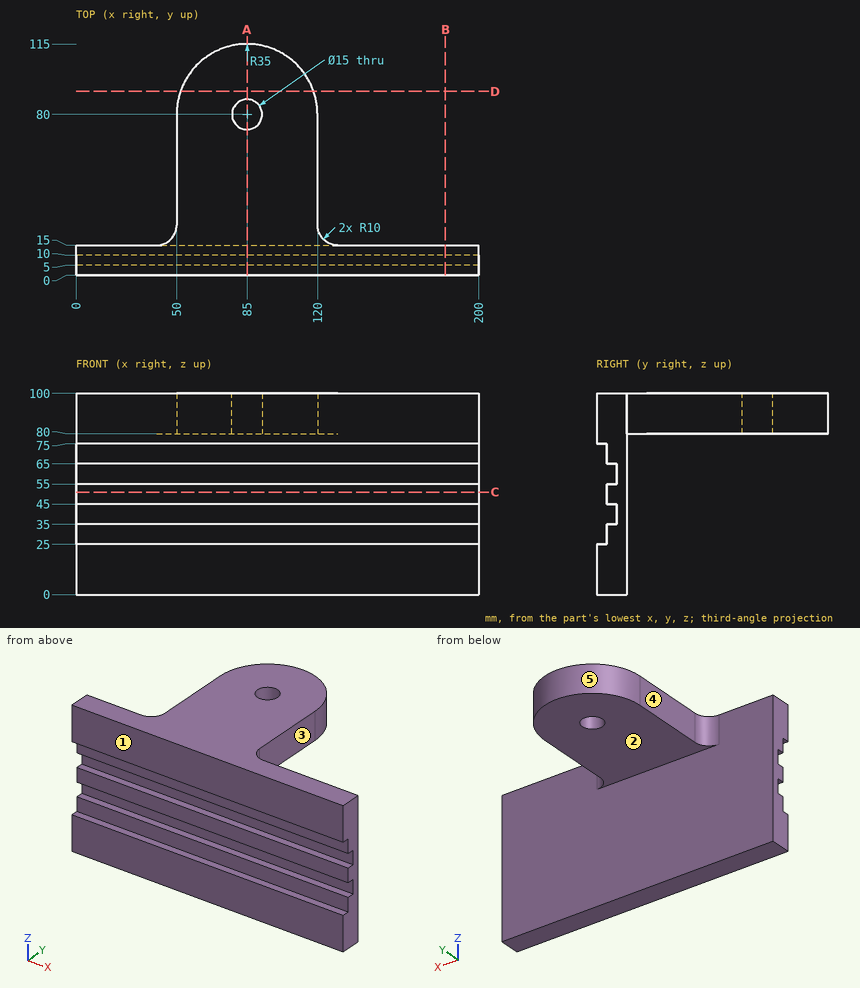
Print and shaded views of the part. All mm, measured from the part's lowest x, y and z. A direction names the side the tool comes from. Round coordinates to 2 decimals unless told otherwise and drop trailing zeros. Write each loop counter-clockwise with the first axis right and the second up, starting at its lowest first coordinate (ties: lowest second). Pieces come first, ordered by that corner, then holes. Notation, with made-up numbers: (2, 72) - (38, 72) arc R22 ccw to (38, 110) - close; hole circle Ø6 at (1, -13). An arc over 180 degrees is marked (long way). Write each question's results on one line, items separated by ' | '. Start each with the question number.
Item 1: Which spindle directions (+Z, -Z, +X, -X, +Y, -Y) get a long thin tool onto all of the face, cutting with end or side? Do the marked faces 1, 2, 3, 4 and 5. Say none if no direction does.
Item 2: Saw through at D-D (y = 91.5). Write the cut outline in (x, z).
Item 3: Drop flat-ended pins along their axis: P1, Ø8, axis at x = 112.5, z = 48.5, coming from the -Y side; P2, Ø8, axis at x = 59, y = 65, coming from the -Z side; P3, Ø10, axis at y = 95, z = 89.5, coming from the +X side. Give the stop position or say it passes through.
Item 4: Wall check: L1, parallel to Y at x = 85, z = 89.25; L2, parallel to Z at x = 66, y = 32; L3, parallel to Y at x = 26.5, z = 67. Give the ranges that are in metal, low to high. Write a range as [from, to].
Item 5: Saw through at C-C (z = 51). Write the cut outline in (x, y), and give its area (3 significant figures).
Item 6: Saw through at B-B (x = 183.5). Write the cut outline in (y, z).
Item 7: Saw through at A-A (x = 85). Write the cut outline in (y, z).
Results are:
1) face 1: +Z, -Z, +X, -X, -Y | face 2: -Z, +X, -X, +Y | face 3: +Z, -Z, +X, +Y | face 4: +Z, -Z, -X, +Y | face 5: +Z, -Z, +Y
2) outline: (51.94, 80) - (118.06, 80) - (118.06, 100) - (51.94, 100) - close
3) P1: stops at y = 5 | P2: stops at z = 80 | P3: stops at x = 118.54
4) L1: y = [0, 72.5], [87.5, 115] | L2: z = [80, 100] | L3: y = [5, 15]
5) outline: (0, 5) - (200, 5) - (200, 15) - (0, 15) - close | area: 2,000 mm²
6) outline: (0, 0) - (15, 0) - (15, 100) - (0, 100) - (0, 75) - (5, 75) - (5, 65) - (10, 65) - (10, 55) - (5, 55) - (5, 45) - (10, 45) - (10, 35) - (5, 35) - (5, 25) - (0, 25) - close
7) outline: (0, 0) - (15, 0) - (15, 80) - (72.5, 80) - (72.5, 100) - (0, 100) - (0, 75) - (5, 75) - (5, 65) - (10, 65) - (10, 55) - (5, 55) - (5, 45) - (10, 45) - (10, 35) - (5, 35) - (5, 25) - (0, 25) - close; (87.5, 80) - (115, 80) - (115, 100) - (87.5, 100) - close
